```python
from build123d import *

# Parameters (mm, degrees)
BOSS_EXTRUDE1_DEPTH       = 400
TAP_DRILL_FOR_8_32_TAP1_D = 3.4544


with BuildPart() as part:
    # Sketch1 → Boss-Extrude1 (new body)
    with BuildSketch(Plane(origin=(0, 0, 0), x_dir=(1, 0, 0), z_dir=(0, 1, 0))):
        Polygon((0, 0), (0, -50.8), (50.8, -50.8), (50.8, 0), (47.625, 0), (47.625, -47.625), (3.175, -47.625), (3.175, 0), align=None)
    extrude(amount=BOSS_EXTRUDE1_DEPTH)

    # Tap Drill for #8-32 Tap1 (through all)
    with Locations(Plane(origin=(50.8, 0, 0), x_dir=(0, 0, -1), z_dir=(1, 0, 0))):
        with Locations((-44.45, 17.3), (-25.4, 17.3), (-6.35, 17.3)):
            Hole(TAP_DRILL_FOR_8_32_TAP1_D / 2)


solid = part.part
```
Check sheet for the modelled part. Datum: model origin and axes. Units: mm. A direction names the side the tool comes from. Give positions to 0.01 mm unless a question says otherwise; leave off trailing zeros. Order: outer loops, then holes, each group sorted by start corner. A loop starts at its lowest first (then second) coordinate and runs counter-clockwise, first axis right, second up. Notation, with made-up numbers: (53.5, 76.5) -> (110.5, 76.5) arc R28 cw to (110.5, 111.5) -> close; hole circle Ø3 at (-15.5, 39.5). An arc over 180 degrees is marked (long way). Return JSON: item names as keys, results as strings.
1. Cross-section at C-C, the plane x = 14. Record the cut outline in (y, z) (3 decimals), plus the area to 3 significant figures.
From the geometry:
{"outline": "(0, 47.625) -> (400, 47.625) -> (400, 50.8) -> (0, 50.8) -> close", "area": "1,270 mm^2"}
2. Material ranges on probe 1 along Z at (x, y) = (1, 17); probe 2 along Y at (x, z) = (2, 25); probe 3 along X at (y, z) = (26.5, 21.5) (3 decimals), recorded low to high. Write a range as [from, to].
From the geometry:
{"probe 1": "[0, 4.65], [8.05, 23.7], [27.1, 42.75], [46.15, 50.8]", "probe 2": "[0, 15.62], [18.98, 400]", "probe 3": "[0, 3.175], [47.625, 50.8]"}
3. Cross-section at A-A, the plane z = 11.5. Record the cut outline in (x, y) (3 decimals), plus the area to 3 significant figures.
From the geometry:
{"outline": "(0, 0) -> (3.175, 0) -> (3.175, 400) -> (0, 400) -> close; (47.625, 0) -> (50.8, 0) -> (50.8, 400) -> (47.625, 400) -> close", "area": "2,540 mm^2"}
4. Mould release check, pull along X, two halves, no side actions. Record for faces 1 (the flat face through (50.8, 197, 26)), 2 (the flat face through (25, 197, 50.8)), 3 (the flat face through (0, 197, 25)), 4 (the flat face through (3.175, 197, 24)): +X half, -X half, draft (parallel to the pull), parting line (faces both ways), or undercut.
From the geometry:
{"face 1": "+X half", "face 2": "draft", "face 3": "-X half", "face 4": "undercut"}
5. Set-up check for faces 5 (the flat face through (26, 197, 47.625)), 6 (the flat face through (25, 0, 48)): record each of +Z, -Z, +X, -X, +Y, -Y from which the full face is reachable in a straight line by a thin tool's end or side.
From the geometry:
{"face 5": "-Z, +Y, -Y", "face 6": "+Z, -Z, +X, -X, -Y"}
6. Cross-section at B-B, the plane y = 194. Record the cut outline in (x, z) (3 decimals), plus the area to 3 significant figures.
From the geometry:
{"outline": "(0, 0) -> (3.175, 0) -> (3.175, 47.625) -> (47.625, 47.625) -> (47.625, 0) -> (50.8, 0) -> (50.8, 50.8) -> (0, 50.8) -> close", "area": "464 mm^2"}
7. Go/stop test with flat-tipped pins: P1, Ø5.5, axis at y = 17.3, z = 6.35, coming from the +X side; P2, Ø8, axis at x = 26.5, y = 268.5, coming from the -Z side (3 decimals). Record where each tip stops, or that it passes through.
From the geometry:
{"P1": "x = 50.8", "P2": "z = 47.625"}
